Autodesk Fusion 360 part; units mm, degrees
sketch "Sketch1" plane through (0, 0, 0) normal (0, 1, 0) x (1, 0, 0)
  circle A0 centre (0, 0) radius 16.5
  dimension "d1" = 33
extrude "Extrude1" add sketch "Sketch1" along normal blind 1
sketch "Sketch2" plane through (0, 1, 0) normal (0, 1, 0) x (-1, 0, 0)
  circle A0 centre (0, 0) radius 16.5
  circle A1 centre (0, 0) radius 13.4
  dimension "d4" = 26.8
extrude "Extrude2" add sketch "Sketch2" along normal blind 2 contours A1
sketch "Sketch3" plane through (0, 3, 0) normal (0, 1, 0) x (-1, 0, 0)
  circle A0 centre (0, 0) radius 13.4
  circle A1 centre (0, 0) radius 11.85
  dimension "d7" = 23.7
extrude "Extrude3" cut sketch "Sketch3" against normal through all contours A1
sketch "Sketch5" plane through (0, 0, 0) normal (1, 0, 0) x (0, 0, -1)
  circle A0 centre (0, 1.36) radius 0.75
  line L0 (16.5, 0) -> (-16.5, 0)
  dimension "d11" = 1.5
  dimension "d12" = 1.36
extrude "Extrude4" cut sketch "Sketch5" along normal through all
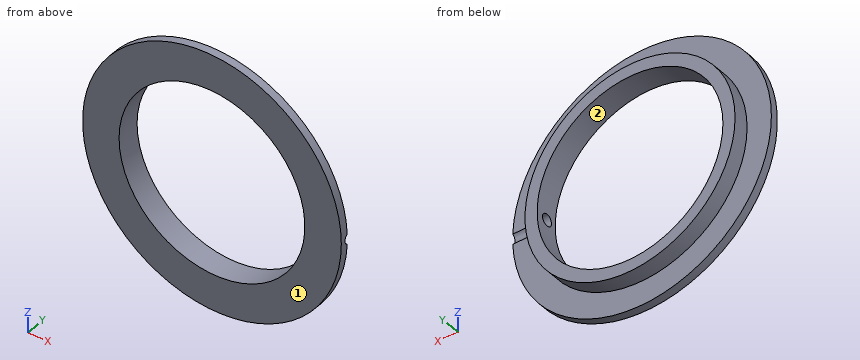
Part model, mm, in its own coordinate system. Face numbers are marked on the shaded views. Round coordinates to 2 decimals unless told otherwise and drop trailing zeros. Write each loop counter-clockwise with the first axis right and the second up, starting at its lowest first coordinate (ties: lowest second). Pieces come first, ordered by that corner, then holes. Notation, with made-up numbers: M 31.5,22.5 L 56.5,22.5 A34 cw 56.5,59.5 Z; hole C 84,18 d3. An arc over 180 degrees is marked long. Return JSON: item names as keys, results as strings. Group by question number.
(1) Two-plate mould, pull along X, no slides. Class the marked faces 1 and 2: +X half, -X half, draft (parallel to the pull), parting line (faces both ways), or undercut.
(2) Saw through at C-C on z = -10. Write the cut outline in (x, y).
(3) Saw through at A-A on x = 7. Write the cut outline in (y, z), then the cut area to 3 significant figures.
(4) Saw through at B-B on z = 0. Write the cut outline in (x, y).
(5) Drill centre lines: probe 1 along X at (y, z) = (2.2, 0); probe 2 along X at (y, z) = (1.95, 0); probe 3 along Y at (x, z) = (-12.5, 7). Where is each one in solid material? Low to high.
(6) Pin check, flat tips, straight feed: pin 1 Ø2 at (x, z) = (-6, -8.5) entering from +Y; pin 2 Ø1.5 at (x, y) = (9, 1.5) entering from +Z; pin 3 Ø16.5 at (x, z) = (3.5, 6) entering from +Y; pin 4 Ø1.5 at (x, z) = (-8, -12.5) entering from +Y. Stop position of each tip, or through.
Returned:
{
 "1": {"face 1": "draft", "face 2": "undercut"},
 "2": {"outline": "M -13.12,0 L -6.36,0 L -6.36,3 L -8.92,3 L -8.92,1 L -13.12,1 Z; M 6.36,0 L 13.12,0 L 13.12,1 L 8.92,1 L 8.92,3 L 6.36,3 Z"},
 "3": {"outline": "M 0,-14.94 L 1,-14.94 L 1,-11.43 L 3,-11.43 L 3,-9.56 L 0,-9.56 Z; M 0,9.56 L 3,9.56 L 3,11.43 L 1,11.43 L 1,14.94 L 0,14.94 Z", "area": "18.2 mm²"},
 "4": {"outline": "M -16.5,0 L -11.85,0 L -11.85,3 L -13.4,3 L -13.4,1 L -16.5,1 Z; M 11.85,0 L 16.5,0 L 16.5,0.61 L 11.85,0.61 Z; M 11.85,2.11 L 13.4,2.11 L 13.4,3 L 11.85,3 Z"},
 "5": {"probe 1": "-13.4 to -11.85, 11.85 to 13.4", "probe 2": "-13.4 to -11.85", "probe 3": "0 to 1"},
 "6": {"pin 1": "through", "pin 2": "z = 14.18", "pin 3": "y = 3", "pin 4": "y = 1"}
}
